```python
from build123d import *

# Parameters (mm, degrees)
EXTRUDE_1_DEPTH          = 18
CHAMFER_1_SIZE           = 5
CHAMFER_2_SIZE           = 5
CUT_EXTRUDE_1_DEPTH      = 8
EXTRUDE_2_REACH          = 696.741
EXTRUDE_2_END_RADIUS     = 240
EXTRUDE_3_DEPTH          = 5
EXTRUDE_4_REACH          = 929.644
EXTRUDE_4_END_RADIUS     = 232
SKETCH_10_R              = 12
CUT_EXTRUDE_7_DEPTH      = 695.872110635
CUT_EXTRUDE_7_DEPTH_BACK = 695.872110635
SKETCH_16_OUTSIDE_W      = 362.68
SKETCH_16_OUTSIDE_H      = 1204.68
SKETCH_16_OUTSIDE_W_2    = 100
SKETCH_16_OUTSIDE_H_2    = 155
SKETCH_21_R              = 1.9
CUT_EXTRUDE_17_DEPTH     = 160.216833407
SKETCH_34_OUTSIDE_W      = 105.66
SKETCH_34_OUTSIDE_H      = 55.66
CUT_EXTRUDE_18_DEPTH     = 40


with BuildPart() as part:
    # Sketch 4 → Loft 1 section 0
    with BuildSketch(Plane(origin=(0, 10, 0), x_dir=(1, 0, 0), z_dir=(0, 1, 0))):
        with BuildLine():
            Line((25, 0), (-25, 0))
            Line((-25, 0), (-25, 630))
            Line((-25, 630), (0, 672.857142857))
            Line((0, 672.857142857), (25, 630))
            Line((25, 630), (25, 0))
        make_face()
    # Sketch 1 → Loft 1 section 1
    with BuildSketch(Plane(origin=(0, 0, 0), x_dir=(1, 0, 0), z_dir=(0, 1, 0))):
        with BuildLine():
            Line((-35, 0), (35, 0))
            Line((35, 0), (35, 630))
            Line((35, 630), (0, 690))
            Line((0, 690), (-35, 630))
            Line((-35, 630), (-35, 0))
        make_face()
    loft_1 = loft()

    # Mirror 1: Loft 1 across plane
    add(loft_1.mirror(Plane.ZX))



with BuildPart() as body_2:
    # Sketch 5 → Extrude 1 (new, symmetric)
    with BuildSketch(Plane(origin=(0, 0, 0), x_dir=(1, 0, 0), z_dir=(0, 1, 0))):
        with BuildLine():
            ThreePointArc((-66.346774613, -65.189169183), (0, -55.5), (66.346774613, -65.189169183))
            ThreePointArc((66.346774613, -65.189169183), (73.061224406, -64.270510235), (76.791165228, -58.612302768))
            ThreePointArc((76.791165228, -58.612302768), (79, -30.5), (76.791165228, -2.387697232))
            ThreePointArc((76.791165228, -2.387697232), (0, -15.004503167), (-76.791165228, -2.387697232))
            ThreePointArc((-76.791165228, -2.387697232), (-79, -30.5), (-76.791165228, -58.612302768))
            ThreePointArc((-76.791165228, -58.612302768), (-73.061224406, -64.270510235), (-66.346774613, -65.189169183))
        make_face()
    extrude(amount=EXTRUDE_1_DEPTH, both=True)

    # Chamfer 1
    chamfer_1_edges = [body_2.edges().sort_by_distance(p)[0] for p in [
        (0, 18, 15.004503167),
        (-79, 18, 30.5),
        (-73.061224406, 18, 64.270510235),
        (0, 18, 55.5),
        (73.061224406, 18, 64.270510235),
        (0, -18, 55.5),
        (-73.061224406, -18, 64.270510235),
        (-79, -18, 30.5),
        (79, -18, 30.5),
        (73.061224406, -18, 64.270510235),
        (79, 18, 30.5),
    ]]
    chamfer(chamfer_1_edges, length=CHAMFER_1_SIZE)

    # Chamfer 2
    chamfer_2_edges = [body_2.edges().sort_by_distance(p)[0] for p in [
        (0, -18, 15.004503167),
    ]]
    chamfer(chamfer_2_edges, length=CHAMFER_2_SIZE)

    # Sketch 6 → Cut-Extrude 1 (cut)
    with BuildSketch(Plane(origin=(0, 18, 0), x_dir=(1, 0, 0), z_dir=(0, 1, 0))):
        with BuildLine():
            ThreePointArc((67.221840199, -55.023712607), (68.932610365, -35.286223394), (68.335500378, -15.483731767))
            ThreePointArc((68.335500378, -15.483731767), (0, -25.004503167), (-68.335500378, -15.483731767))
            ThreePointArc((-68.335500378, -15.483731767), (-68.932610365, -35.286223394), (-67.221840199, -55.023712607))
            ThreePointArc((-67.221840199, -55.023712607), (0, -45.5), (67.221840199, -55.023712607))
        make_face()
    cut_extrude_1 = extrude(amount=-CUT_EXTRUDE_1_DEPTH, mode=Mode.SUBTRACT)

    # Mirror 2: Cut-Extrude 1 across plane
    add(cut_extrude_1.mirror(Plane.ZX), mode=Mode.SUBTRACT)


with BuildPart() as part_1:
    add(part.part)

    add(body_2.part)  # Extrude 2 merges body 2
    # Extrude 2: up to this cylinder (the profile starts inside it)
    extrude_2_end = Plane(origin=(0, 0, -224.995496833), z_dir=(0, -1, 0)) * Cylinder(EXTRUDE_2_END_RADIUS, 1874.482, mode=Mode.PRIVATE)
    # Sketch 7 → Extrude 2 (add, up to the surface)
    with BuildSketch(Plane.XY, mode=Mode.PRIVATE) as extrude_2_sk1:
        Polygon((-25.828427125, 12), (-37.828427125, 0), (-25.828427125, -12), (25.828427125, -12), (37.828427125, 0), (25.828427125, 12), align=None)
    extrude_2_tool1 = extrude(extrude_2_sk1.sketch, amount=EXTRUDE_2_REACH, mode=Mode.PRIVATE) & extrude_2_end
    add(extrude_2_tool1.solids().sort_by_distance((0, 0, 0))[0])

    # Sketch 8 → Extrude 3 (add)
    with BuildSketch(Plane(origin=(0, 0, 0), x_dir=(-1, 0, 0), z_dir=(0, 0, -1))):
        Polygon((25.828427125, 12), (-25.828427125, 12), (-37.828427125, 0), (-25.828427125, -12), (25.828427125, -12), (37.828427125, 0), align=None)
    extrude(amount=EXTRUDE_3_DEPTH)



with BuildPart() as body_2_2:
    # Sketch 9 → Revolve 1 (revolve)
    with BuildSketch(Plane(origin=(0, 0, 0), x_dir=(1, 0, 0), z_dir=(0, 1, 0))):
        Polygon((0, -310), (0, -234), (-12, -234), (-22.5, -256), align=None)
    revolve(axis=Axis((0, 0, -690), (0, 0, 1)))


with BuildPart() as part_2:
    add(part_1.part)

    add(body_2_2.part)  # Extrude 4 merges body 2 2
    # Extrude 4: up to this cylinder (the profile starts inside it)
    extrude_4_end = Plane(origin=(0, 0, 287.5), z_dir=(0, -1, 0)) * Cylinder(EXTRUDE_4_END_RADIUS, 2324.288, mode=Mode.PRIVATE)
    # Sketch 10 → Extrude 4 (add, up to the surface)
    with BuildSketch(Plane(origin=(0, 0, 234), x_dir=(-1, 0, 0), z_dir=(0, 0, -1)), mode=Mode.PRIVATE) as extrude_4_sk1:
        with Locations(Location((0, 0, 0), (0, 0, 90))):
            Circle(SKETCH_10_R)
    extrude_4_tool1 = extrude(extrude_4_sk1.sketch, amount=EXTRUDE_4_REACH, mode=Mode.PRIVATE) & extrude_4_end
    add(extrude_4_tool1.solids().sort_by_distance((0, 0, 234))[0])

    # Sketch 16 outside → Cut-Extrude 7 (cut, two sides: drawn at the far end of the back side and taken through both)
    with BuildSketch(Plane(origin=(0, 0, 0), x_dir=(1, 0, 0), z_dir=(0, 1, 0)).offset(-CUT_EXTRUDE_7_DEPTH_BACK)):
        with Locations((0, 190)):
            Rectangle(SKETCH_16_OUTSIDE_W, SKETCH_16_OUTSIDE_H)
        with Locations((0, 612.5)):
            Rectangle(SKETCH_16_OUTSIDE_W_2, SKETCH_16_OUTSIDE_H_2, mode=Mode.SUBTRACT)
    extrude(amount=CUT_EXTRUDE_7_DEPTH + CUT_EXTRUDE_7_DEPTH_BACK, mode=Mode.SUBTRACT)

    # Sketch 21 → Cut-Extrude 17 (cut, through all)
    with BuildSketch(Plane.XY.offset(-535)):
        Circle(SKETCH_21_R)
    extrude(amount=-CUT_EXTRUDE_17_DEPTH, mode=Mode.SUBTRACT)

    # Sketch 34 outside → Cut-Extrude 18 (cut)
    with BuildSketch(Plane.XY.offset(-535)):
        Rectangle(SKETCH_34_OUTSIDE_W, SKETCH_34_OUTSIDE_H)
        Polygon((-22.928932188, -5), (22.928932188, -5), (27.928932188, 0), (22.928932188, 5), (-22.928932188, 5), (-27.928932188, 0), align=None, mode=Mode.SUBTRACT)
    extrude(amount=-CUT_EXTRUDE_18_DEPTH, mode=Mode.SUBTRACT)


solid = part_2.part
```
Source: CAD feature listing. Evaluate the final solid. Frame: model axes, mm. A direction names the side the tool comes from. Coordinates: 2 decimals unless noted, no trailing zeros. Write each loop counter-clockwise with the first axis right and the second up, starting at its lowest first coordinate (ties: lowest second). Pieces come first, ordered by that corner, then holes. Notation, with made-up numbers: (18.25, 1) - (24.25, 1) arc R5 ccw to (24.25, 6) - close; hole circle Ø1 at (66, 8.25). An arc over 180 degrees is marked (long way). Answer as a JSON object with one key per item and string values.
Q1. Material intervals for line 1 (X direction, y = 0, z = -588); line 2 (Y direction, x = 0, z = -651); line 3 (Y direction, x = 0, z = -567), sorted ascending. Write a range as [from, to].
Ans:
{"line 1": "x = [-35, -1.9], [1.9, 35]", "line 2": "y = [-10, -1.9], [1.9, 10]", "line 3": "y = [-5, -1.9], [1.9, 5]"}
Q2. Set-up query: faces 1 (the flat face through (0, 5, -555)), 2 (the flat face through (-25.394, 2.535, -554.72)), 3 (the flat face through (-25.46, -2.47, -554.72)). Return all of +Z, -Z, +X, -X, +Y, -Y with unobstructed straight access to the full face (end or side cutting, diameter ignored); none if empty.
Ans:
{"face 1": "+Z, +X, -X, +Y", "face 2": "+Z, -X, +Y", "face 3": "+Z, -X, -Y"}
Q3. First-contact query: pin 1 Ø4 at (x, y) = (-27, 6.5) entering from -Z; pin 2 Ø4 at (x, z) = (-11, -564) entering from -Y; pin 3 Ø2 at (x, z) = (13.5, -657) entering from +Y. Flat tips, straight axial feed; report the tip coordinate or a pass-through.
Ans:
{"pin 1": "stops at z = -637.42", "pin 2": "stops at y = -5", "pin 3": "stops at y = 6.91"}
Q4. Section query A-A, the plane z = -618.5. Output: boundary loops of the cut face in (x, y), plus the area to 3 significant figures.
Ans:
{"outline": "(-35, 0) - (-25, -10) - (25, -10) - (35, 0) - (25, 10) - (-25, 10) - close; hole circle Ø3.8 at (0, 0)", "area": "1,190 mm2"}
